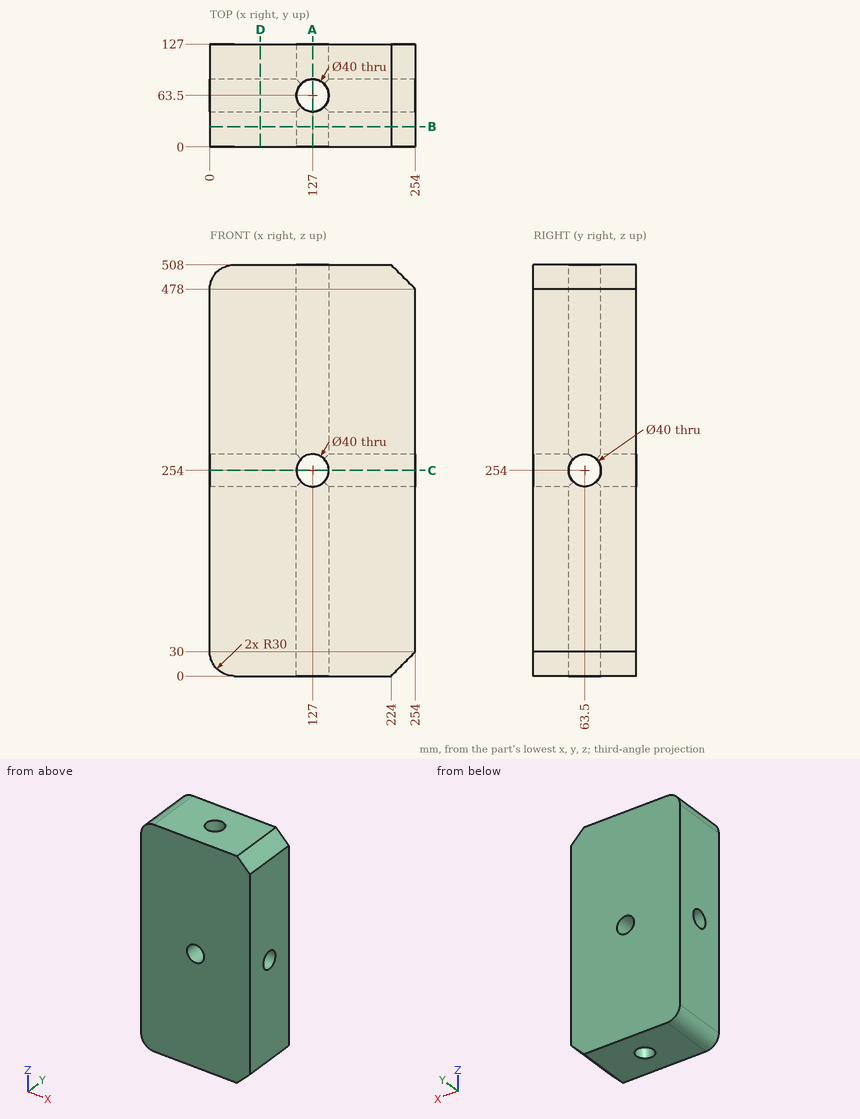
Geometry: see drawing. Coordinates: mm, zero at the bounding-box minimum. Give positions to 0.01 mm unless a question says otherwise; leave off trailing zeros. Loops run counter-clockwise (first coordinate to the right, second up) from the corner with the lowest first, then second, coordinate; pieces in that order, holes last. Notation, with made-up numbers: (72.25, 46.5) - (131.25, 46.5) arc R15 ccw to (131.25, 52.5) - close; hole circle Ø1 at (-7, -30.75). An arc over 180 degrees is marked (long way). Use CSV: the item, a comma, the result in double quotes. Start each with the question number.
1. Section C-C (z = 254). Output: boundary loops of the cut face in (x, y), then the cut area to 3 significant figures.
2. Section D-D (x = 62.5). Output: boundary loops of the cut face in (y, z).
3. Ray query, L1, parallel to Z at x = 127, y = 99.5; L2, parallel to X at y = 63, z = 456; L3, parallel to Y at x = 127, z = 164.5. Return the intervals inside material, ascending.
4. Pin query (flat end, axial travel): pin 1 (24 mm diameter, centred on x = 127, y = 63.5, fed in from +Z). Return the tip coordinate at first contact, or that it passes through.
5. Section B-B (y = 25). Output: boundary loops of the cut face in (x, z).
6. Section A-A (x = 127). Output: boundary loops of the cut face in (y, z).
Response:
1,outline,"(0, 0) - (107, 0) - (107, 43.5) - (0, 43.5) - close; (0, 83.5) - (107, 83.5) - (107, 127) - (0, 127) - close; (147, 0) - (254, 0) - (254, 43.5) - (147, 43.5) - close; (147, 83.5) - (254, 83.5) - (254, 127) - (147, 127) - close"
1,area,"18,600 mm²"
2,outline,"(0, 0) - (127, 0) - (127, 508) - (0, 508) - close; hole circle Ø40 at (63.5, 254)"
3,L1,"0 to 234, 274 to 508"
3,L2,"0 to 107.01, 146.99 to 254"
3,L3,"0 to 43.5, 83.5 to 127"
4,pin 1,"through"
5,outline,"(0, 30) arc R30 ccw to (30, 0) - (224, 0) - (254, 30) - (254, 478) - (224, 508) - (30, 508) arc R30 ccw to (0, 478) - close; hole circle Ø40 at (127, 254)"
6,outline,"(0, 0) - (43.5, 0) - (43.5, 234) - (0, 234) - close; (0, 274) - (43.5, 274) - (43.5, 508) - (0, 508) - close; (83.5, 0) - (127, 0) - (127, 234) - (83.5, 234) - close; (83.5, 274) - (127, 274) - (127, 508) - (83.5, 508) - close"
